Check sheet for the modelled part. Datum: model origin and axes. Units: mm. Give positions to 0.01 mm unless a question says otherwise; leave off trailing zeros. Order: outer loops, then holes, each group sorted by start corner. A loop starts at its lowest first (then second) coordinate and runs counter-clockwise, first axis right, second up.
from build123d import *

# Parameters (mm, degrees)
SKETCH1_W           = 5.08
SKETCH1_H           = 20.955
SKETCH1_H_2         = 22.098
BOSS_EXTRUDE1_DEPTH = 3.175


with BuildPart() as part:
    # Sketch1 → Boss-Extrude1 (new body)
    with BuildSketch(Plane(origin=(0, 0, 0), x_dir=(1, 0, 0), z_dir=(0, 1, 0))):
        with BuildLine():
            Line((36.195, 27.94), (36.195, 22.098))
            ThreePointArc((36.195, 22.098), (35.823025612, 21.199974388), (34.925, 20.828))
            Line((34.925, 20.828), (-17.145, 20.828))
            ThreePointArc((-17.145, 20.828), (-18.043025612, 21.199974388), (-18.415, 22.098))
            Line((-18.415, 22.098), (-18.415, 27.94))
            Line((-18.415, 27.94), (-22.4282, 27.94))
            Line((-22.4282, 27.94), (-22.4282, 31.623))
            ThreePointArc((-22.4282, 31.623), (-22.800174388, 32.521025612), (-23.6982, 32.893))
            Line((-23.6982, 32.893), (-33.0454, 32.893))
            ThreePointArc((-33.0454, 32.893), (-33.943425612, 32.521025612), (-34.3154, 31.623))
            Line((-34.3154, 31.623), (-34.3154, 27.94))
            Line((-34.3154, 27.94), (-42.799, 27.94))
            Line((-42.799, 27.94), (-42.799, -27.94))
            Line((-42.799, -27.94), (-34.3154, -27.94))
            Line((-34.3154, -27.94), (-34.3154, -31.623))
            ThreePointArc((-34.3154, -31.623), (-33.943425612, -32.521025612), (-33.0454, -32.893))
            Line((-33.0454, -32.893), (-23.6982, -32.893))
            ThreePointArc((-23.6982, -32.893), (-22.800174388, -32.521025612), (-22.4282, -31.623))
            Line((-22.4282, -31.623), (-22.4282, -27.94))
            Line((-22.4282, -27.94), (36.195, -27.94))
            Line((36.195, -27.94), (36.195, -29.718))
            Line((36.195, -29.718), (39.37, -29.718))
            Line((39.37, -29.718), (39.37, -27.94))
            Line((39.37, -27.94), (42.799, -27.94))
            Line((42.799, -27.94), (42.799, 27.94))
            Line((42.799, 27.94), (39.37, 27.94))
            Line((39.37, 27.94), (39.37, 29.718))
            Line((39.37, 29.718), (36.195, 29.718))
            Line((36.195, 29.718), (36.195, 27.94))
        make_face()
        with Locations((37.719, -0.7493)):
            Rectangle(SKETCH1_W, SKETCH1_H, mode=Mode.SUBTRACT)
        with Locations((-2.54, -15.875)):
            Rectangle(SKETCH1_W, SKETCH1_H_2, mode=Mode.SUBTRACT)
    extrude(amount=BOSS_EXTRUDE1_DEPTH)


solid = part.part
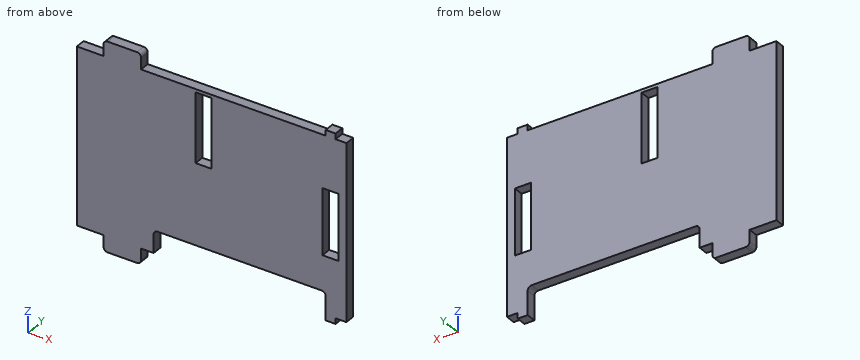
1) Section check C-C, the plane y = 1.15. State how many separate pieces and enclosed holes the cut face has, then the cut area to 3 significant figures.
Recorded:
separate pieces: 1
enclosed holes: 2
area: 4,300 mm2
2) Section check D-D, the plane x = 25. Record the cut outline in (y, z) (3 decimals), then the cut area to 3 significant figures.
Recorded:
outline: (0, -20.828) - (3.175, -20.828) - (3.175, 27.94) - (0, 27.94) - close
area: 155 mm2
3) Section check B-B, the plane z = -24. Record the cut outline in (x, y) (3 decimals).
Recorded:
outline: (-42.799, 0) - (-18.415, 0) - (-18.415, 3.175) - (-42.799, 3.175) - close; (36.195, 0) - (42.799, 0) - (42.799, 3.175) - (36.195, 3.175) - close
4) Depth check by flat-ended pin: pin 1 Ø1 at (x, y) = (37, 2) entering from -Z; pin 2 Ø1.4 at (y, z) = (2, -29) entering from +X; pin 3 Ø1.4 at (y, z) = (2, 29) entering from -X. Enter the tip coordinate at first touch or a pass-through.
Recorded:
pin 1: stops at z = -29.72
pin 2: stops at x = 39.37
pin 3: stops at x = -34.32
5) Material ranges on L1, parallel to X at y = 0.75, z = 8; L2, parallel to X at y = 0.85, z = 19; L3, parallel to Z at x = -4.5, y = 0.2, recorded low to high.
Recorded:
L1: x = -42.8 to -5.08, 0 to 35.18, 40.26 to 42.8
L2: x = -42.8 to -5.08, 0 to 42.8
L3: z = -20.83 to 4.83, 26.92 to 27.94
6) Section check A-A, the plane x = -2. Record the cut outline in (y, z) (3 decimals).
Recorded:
outline: (0, -20.828) - (3.175, -20.828) - (3.175, 4.826) - (0, 4.826) - close; (0, 26.924) - (3.175, 26.924) - (3.175, 27.94) - (0, 27.94) - close
